The model under review builds one solid part; all positions refer to its coordinate system, in mm. A direction names the side the tool comes from. Coordinates: 2 decimals unless noted, no trailing zeros. Write each loop counter-clockwise with the first axis right and the second up, starting at its lowest first coordinate (ties: lowest second). Pieces come first, ordered by that corner, then holes.
1) For P1, Ø1.2, axis at y = 0, z = 7, coming from the -X side; P2, Ø8, axis at y = 12, z = 11.5, coming from the +X side; P3, Ø1.7, axis at y = 16, z = 11.67, coming from the -X side, all flat-tipped, find the tip position at first contact; note any pin that passes through.
2) Mouldability with a two-part tool opening along Y and no side actions: class faces 4 (the flat face through (-4.5, 0, 5)), 5 (the flat face through (0, 19, -2)), 6 (the cylindrical face through (-0.021, 16.553, 12.174)) as released by +Y, released by -Y, zero draft, split by the parting line, or undercut.
3) Add section B-B, the plane z = 5. State the section outline as (x, y) points.
4) Add section C-C, the plane x = 2. State the section outline as (y, z) points.
5) Machinability: for faces 1 (the flat face through (-1.5, 8, 5)), 2 (the flat face through (1.5, -1, 5)), 3 (the flat face through (-0.1, 0.5, 10)), which of the approach directions +Z, -Z, +X, -X, +Y, -Y give a long, thin tool a straight path to every point of the face, cutting with its end or side? Answer none if there is none.
6) For line 1 (Z direction, x = 0.6, y = 16); line 2 (X direction, y = 10.5, z = 9); line 3 (Y direction, x = 4.25, z = 6.75), list the stretches that pass through material, from the lowest coordinate up.
7) Add section D-D, the plane y = 12.5. State the section outline as (x, z) points, then the cut area to 3 significant figures.
8) Add section A-A, the plane y = 16. State the section outline as (x, z) points.
from build123d import *

# Parameters (mm, degrees)
BOSS_EXTRUDE1_DEPTH = 10
SKETCH2_W           = 10
SKETCH2_H           = 16.666666666
BOSS_EXTRUDE2_DEPTH = 2
SKETCH3_W           = 3
SKETCH3_H           = 15
BOSS_EXTRUDE3_DEPTH = 16.666666667
CUT_EXTRUDE1_DEPTH  = 25.104517788
SKETCH5_R           = 0.75
CUT_EXTRUDE2_DEPTH  = 25.104517788


with BuildPart() as part:
    # Sketch1 → Boss-Extrude1 (new body)
    with BuildSketch(Plane.XY):
        Polygon((-1.5, -2), (-1.5, 0), (1.5, 0), (1.5, -2), (4.5, -2), (4.5, 2), (-4.5, 2), (-4.5, -2), align=None)
    extrude(amount=BOSS_EXTRUDE1_DEPTH)

    # Sketch2 → Boss-Extrude2 (add)
    with BuildSketch(Plane(origin=(0, 2, 0), x_dir=(1, 0, 0), z_dir=(0, 1, 0))):
        with Locations((0, -5)):
            Rectangle(SKETCH2_W, SKETCH2_H)
    extrude(amount=BOSS_EXTRUDE2_DEPTH)

    # Sketch3 → Boss-Extrude3 (add)
    with BuildSketch(Plane.XY.offset(13.333333333)):
        with Locations((0, 11.5)):
            Rectangle(SKETCH3_W, SKETCH3_H)
    extrude(amount=-BOSS_EXTRUDE3_DEPTH)

    # Sketch4 → Cut-Extrude1 (cut, through all)
    with BuildSketch(Plane.ZY.offset(1.5)):
        with BuildLine():
            Line((0, 14), (0, 19))
            Line((0, 19), (10, 19))
            Line((10, 19), (10, 14))
            ThreePointArc((10, 14), (5, 9), (0, 14))
        make_face()
    extrude(amount=-CUT_EXTRUDE1_DEPTH, mode=Mode.SUBTRACT)

    # Sketch5 → Cut-Extrude2 (cut, through all)
    with BuildSketch(Plane.ZY.offset(1.5)):
        with Locations(Location((11.666666667, 16, 0), (0, 0, 270))):
            Circle(SKETCH5_R)
        with Locations(Location((-1.666666667, 16, 0), (0, 0, 270))):
            Circle(SKETCH5_R)
    extrude(amount=-CUT_EXTRUDE2_DEPTH, mode=Mode.SUBTRACT)


solid = part.part
Geometry results:
1. P1: stops at x = -4.5
1. P2: stops at x = 1.5
1. P3: stops at x = -1.5
2. face 4: zero draft
2. face 5: released by +Y
2. face 6: undercut
3. outline: (-5, 2) - (-4.5, 2) - (-4.5, -2) - (-1.5, -2) - (-1.5, 0) - (1.5, 0) - (1.5, -2) - (4.5, -2) - (4.5, 2) - (5, 2) - (5, 4) - (1.5, 4) - (1.5, 9) - (-1.5, 9) - (-1.5, 4) - (-5, 4) - close
4. outline: (-2, 0) - (2, 0) - (2, -3.33) - (4, -3.33) - (4, 13.33) - (2, 13.33) - (2, 10) - (-2, 10) - close
5. face 1: +Z, -Z, -X, +Y
5. face 2: +Z, -Z, -Y
5. face 3: +Z, +X, -X, -Y
6. line 1: z = -3.33 to -2.42, -0.92 to 0, 10 to 10.92, 12.42 to 13.33
6. line 2: x = -1.5 to 1.5
6. line 3: y = -2 to 4
7. outline: (-1.5, -3.33) - (1.5, -3.33) - (1.5, 0.23) - (-1.5, 0.23) - close; (-1.5, 9.77) - (1.5, 9.77) - (1.5, 13.33) - (-1.5, 13.33) - close
7. area: 21.4 mm2
8. outline: (-1.5, -3.33) - (1.5, -3.33) - (1.5, -2.42) - (-1.5, -2.42) - close; (-1.5, -0.92) - (1.5, -0.92) - (1.5, 0) - (-1.5, 0) - close; (-1.5, 10) - (1.5, 10) - (1.5, 10.92) - (-1.5, 10.92) - close; (-1.5, 12.42) - (1.5, 12.42) - (1.5, 13.33) - (-1.5, 13.33) - close
